from build123d import *

# Parameters (mm, degrees)
SKETCH_1_W          = 160
SKETCH_1_H          = 96
SKETCH_1_R          = 4
SKETCH_1_W_2        = 140
SKETCH_1_H_2        = 48
EXTRUDE_1_DEPTH     = 25
FILLET_1_R          = 30
FILLET_2_R          = 5
SKETCH_11_R         = 6.498169544
SKETCH_11_R_2       = 6.5
CUT_EXTRUDE_1_DEPTH = 15


with BuildPart() as part:
    # 草图1 → 凸台-拉伸1 (new body)
    with BuildSketch(Plane(origin=(0, 0, 0), x_dir=(0, 0, -1), z_dir=(1, 0, 0))):
        with Locations((18.05845234, 14.323348887)):
            Rectangle(SKETCH_1_W, SKETCH_1_H)
        with Locations((-2.443633142, 46.063348887)):
            Circle(SKETCH_1_R, mode=Mode.SUBTRACT)
        with Locations((37.163019963, 46.063348887)):
            Circle(SKETCH_1_R, mode=Mode.SUBTRACT)
        with Locations((-2.443633142, -16.944440743)):
            Circle(SKETCH_1_R, mode=Mode.SUBTRACT)
        with Locations((37.163019963, -16.944440743)):
            Circle(SKETCH_1_R, mode=Mode.SUBTRACT)
        with Locations((64.784581693, 46.063348887)):
            Circle(SKETCH_1_R, mode=Mode.SUBTRACT)
        with Locations((-30.063633142, -16.944440743)):
            Circle(SKETCH_1_R, mode=Mode.SUBTRACT)
        with Locations((64.784581693, -16.944440743)):
            Circle(SKETCH_1_R, mode=Mode.SUBTRACT)
        with Locations((-30.063633142, 46.063348887)):
            Circle(SKETCH_1_R, mode=Mode.SUBTRACT)
        with Locations((18.05845234, 14.323348887)):
            Rectangle(SKETCH_1_W_2, SKETCH_1_H_2, mode=Mode.SUBTRACT)
    extrude(amount=-EXTRUDE_1_DEPTH)

    # 圆角1
    fillet_1_edges = [part.edges().sort_by_distance(p)[0] for p in [
        (-12.5, 62.323348887, 61.94154766),
        (-12.5, 62.323348887, -98.05845234),
        (-12.5, -33.676651113, -98.05845234),
        (-12.5, -33.676651113, 61.94154766),
    ]]
    fillet(fillet_1_edges, radius=FILLET_1_R)

    # 圆角2
    fillet_2_edges = [part.edges().sort_by_distance(p)[0] for p in [
        (-12.5, -9.676651113, 51.94154766),
        (-12.5, 38.323348887, 51.94154766),
        (-12.5, 38.323348887, -88.05845234),
        (-12.5, -9.676651113, -88.05845234),
    ]]
    fillet(fillet_2_edges, radius=FILLET_2_R)

    # 草图11 → 切除-拉伸1 (cut)
    with BuildSketch(Plane(origin=(0, 0, 0), x_dir=(0, 0, -1), z_dir=(1, 0, 0))):
        with Locations((37.163019963, 46.063348887)):
            Circle(SKETCH_11_R)
        with Locations((-2.443633142, 46.063348887)):
            Circle(SKETCH_11_R_2)
        with Locations((37.163019963, -16.944440743)):
            Circle(SKETCH_11_R_2)
        with Locations((-2.443633142, -16.944440743)):
            Circle(SKETCH_11_R_2)
    extrude(amount=-CUT_EXTRUDE_1_DEPTH, mode=Mode.SUBTRACT)


solid = part.part
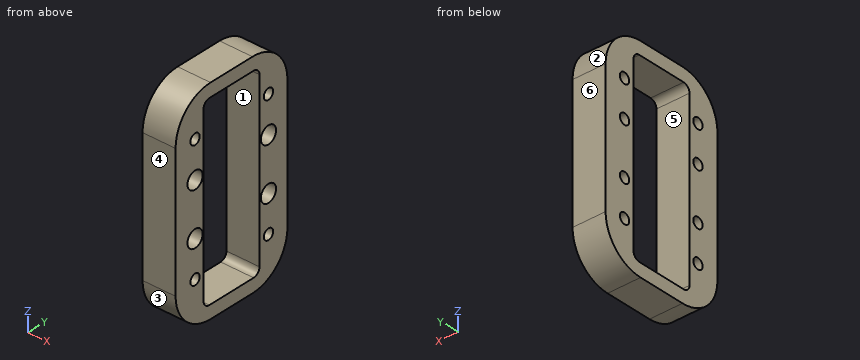
Can you work these out from the model? Positions are in its coordinate system, mm. Face numbers are marked on the shaded views. A direction names the side the tool comes from. Round coordinates to 2 decimals unless told otherwise and drop trailing zeros. Loops run counter-clockwise (first coordinate to the right, second up) from the corner with the lowest first, then second, coordinate; pieces in that order, holes last. Notation, with made-up numbers: (-35, 64) - (-31, 64) arc R11 ccw to (-31, 75) - close; hole circle Ø9 at (-14.75, 4.5). An arc over 180 degrees is marked (long way). Answer in a Markdown table with one row per item. Add a question column.
Q1. For pin 1 Ø5 at (x, y) = (-7.5, 47.5) entering from +Z; pin 2 Ø1.5 at (x, z) = (-13, 34) entering from +Y, each with a flat end and sliding along its axis, tell me the tip position at first contact or that it passes through.
Q2. Which directions (+Z, -Z, +X, -X, +Y, -Y) give clear straight access to the entire face, cutting with the end or side of a thin tool? Please do the marked faces 5 and 6.
Q3. I want a section at C-C on x = -21. Count the separate pieces of the cut face and the enclosed holes in it, and give its area (3 significant figures).
Q4. I want a section at B-B on y = 25.5. List the corners of the cut face in (x, z) for me.
Q5. I want a section at D-D on z = -66. List the corners of the cut face in (x, y) for me, and give its area (3 significant figures).
Q6. We'd pull the mould along Z, two halves only. Please class the marked faces 1, 2, 3 and 4: pulls with the +Z half, pulls with the -Z half, needs draft (parallel to the pull), parting line crosses it, or undercut.
Q7. I want a section at A-A on z = -11.5. List the corners of the cut face in (x, y) for me.
Q8. I need wall thicknesses on L1, parallel to Y at x = -19.25, z = 30.5; L2, parallel to Z at x = -6.5, y = 17; L3, parallel to Y at x = -2.5, z = -8. Which ranges of each line are inside material? Lowest first, please.
A:
| question | item | result |
|---|---|---|
| 1 | pin 1 | z = 59.13 |
| 1 | pin 2 | y = 62.29 |
| 2 | face 5 | +X, -X |
| 2 | face 6 | +Z, -Z, +X, -X, +Y |
| 3 | separate pieces | 1 |
| 3 | enclosed holes | 9 |
| 3 | area | 7,490 mm^2 |
| 4 | outline | (-25, -98.06) - (0, -98.06) - (0, -88.06) - (-25, -88.06) - close; (-25, 51.94) - (0, 51.94) - (0, 61.94) - (-25, 61.94) - close |
| 5 | outline | (-25, -33.68) - (0, -33.68) - (0, -20.76) - (-25, -20.76) - close; (-25, -13.13) - (0, -13.13) - (0, -9.68) - (-25, -9.68) - close; (-25, 38.32) - (0, 38.32) - (0, 42.25) - (-25, 42.25) - close; (-25, 49.87) - (0, 49.87) - (0, 62.32) - (-25, 62.32) - close |
| 5 | area | 819 mm^2 |
| 6 | face 1 | undercut |
| 6 | face 2 | pulls with the +Z half |
| 6 | face 3 | pulls with the -Z half |
| 6 | face 4 | needs draft |
| 7 | outline | (-25, -33.68) - (0, -33.68) - (0, -9.68) - (-25, -9.68) - close; (-25, 38.32) - (0, 38.32) - (0, 62.32) - (-25, 62.32) - close |
| 8 | L1 | -33.68 to -20.92, -12.97 to -9.68, 38.32 to 42.09, 50.04 to 62.32 |
| 8 | L2 | -98.06 to -88.06, 51.94 to 61.94 |
| 8 | L3 | -33.68 to -9.68, 38.32 to 62.32 |
